Geometry: see drawing. Coordinates: mm, zero at the bounding-box minimum. Give positions to 0.01 mm unless a question says otherwise; leave off trailing zeros. Write each loop counter-clockwise with the first axis right and the second up, starting at its lowest first coordinate (ties: lowest second). Pieces come first, ordered by that corner, then holes. Notation, with made-up numbers: (66.25, -21.75) -> (78.25, -21.75) arc R8 ccw to (78.25, -16.75) -> close; hole circle Ø7 at (-35.75, -1.5). An arc over 180 degrees is marked (long way). Answer as a JSON object with one key per item and string values. Group by question number.
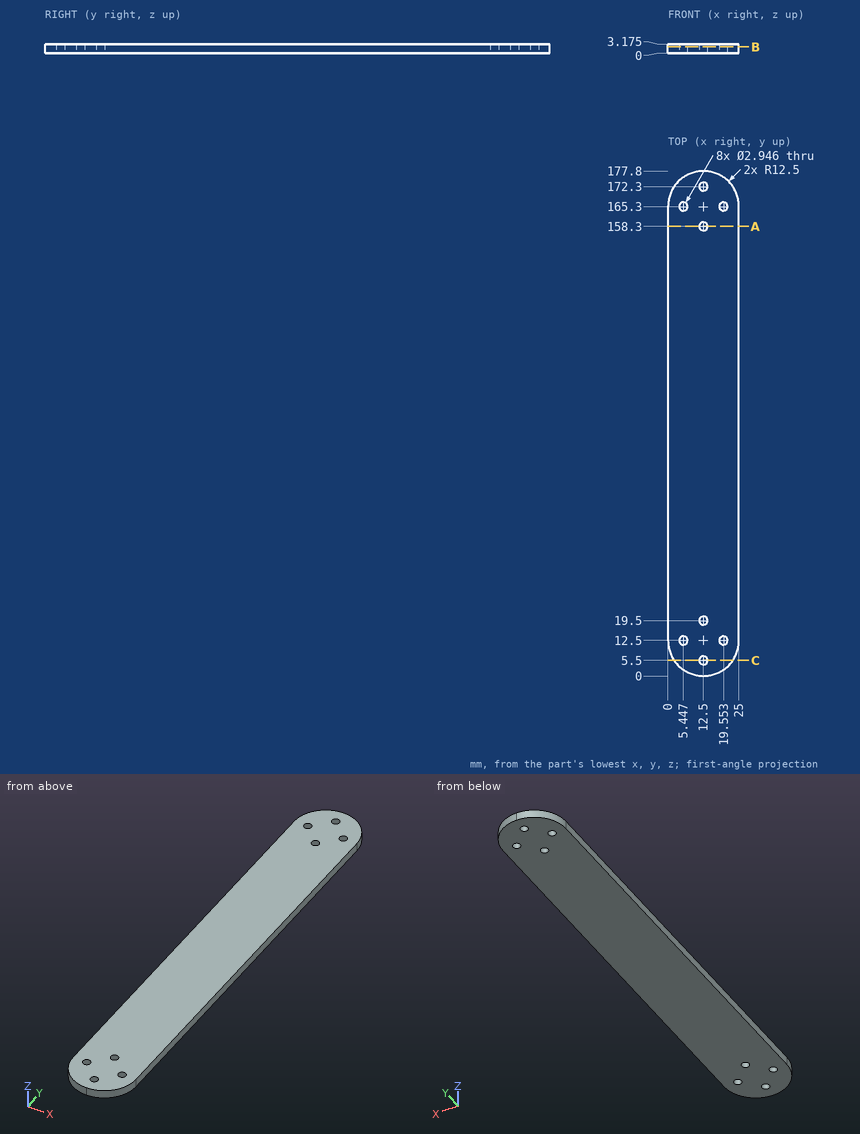
1. Section B-B (z = 2.2). State how many separate pieces and enclosed holes the cut face has, plus the area to 3 significant figures.
2. Contact query for flat-ended pins moving along their axis: pin 1 Ø2 at (x, y) = (8, 143.5) entering from -Z; pin 2 Ø2.5 at (x, y) = (5.45, 165.3) entering from -Z. Output: stop coordinate, or through.
3. Section C-C (y = 5.5). Return the cut outline in (x, z) (1 decimal), plus the area to 3 significant figures.
4. Section A-A (y = 158.3). Return the cut outline in (x, z) (1 decimal).
5. Line query: line 1 (Y direction, x = 11.75, z = 0.7); line 2 (Y direction, x = 18.5, z = 1.45) (1 decimal); line 3 (Y direction, x = 11.5, z = 0.9). Output: solid intervals per line, ascending.
Working result:
{
 "1": {"separate pieces": "1", "enclosed holes": "8", "area": "4,260 mm^2"},
 "2": {"pin 1": "stops at z = 0", "pin 2": "passes through"},
 "3": {"outline": "(2.1, 0) -> (11, 0) -> (11, 3.2) -> (2.1, 3.2) -> close; (14, 0) -> (22.9, 0) -> (22.9, 3.2) -> (14, 3.2) -> close", "area": "56.4 mm^2"},
 "4": {"outline": "(0, 0) -> (11, 0) -> (11, 3.2) -> (0, 3.2) -> close; (14, 0) -> (25, 0) -> (25, 3.2) -> (14, 3.2) -> close"},
 "5": {"line 1": "y = 0.02 to 4.23, 6.77 to 18.23, 20.77 to 157.03, 159.57 to 171.03, 173.57 to 177.78", "line 2": "y = 1.5 to 11.5, 13.5 to 164.3, 166.3 to 176.3", "line 3": "y = 0.04 to 4.42, 6.58 to 18.42, 20.58 to 157.22, 159.38 to 171.22, 173.38 to 177.76"}
}
